For this review, use the dimensioned drawing (mm, ordinates from the lowest corner) and the shaded views. A direction names the side the tool comes from. Give positions to 0.01 mm unless a question says otherwise; leave off trailing zeros. Order: outer loops, then holes, each group sorted by start corner. A loop starts at its lowest first (then second) coordinate and runs counter-clockwise, first axis right, second up. Notation, with made-up numbers: (30.25, 58.5) -> (85.25, 58.5) arc R22 cw to (85.25, 67.5) -> close; hole circle Ø9 at (85.5, 85). An arc over 180 degrees is marked (long way). Answer as a JSON object with one key per item and string values. Group by question number.
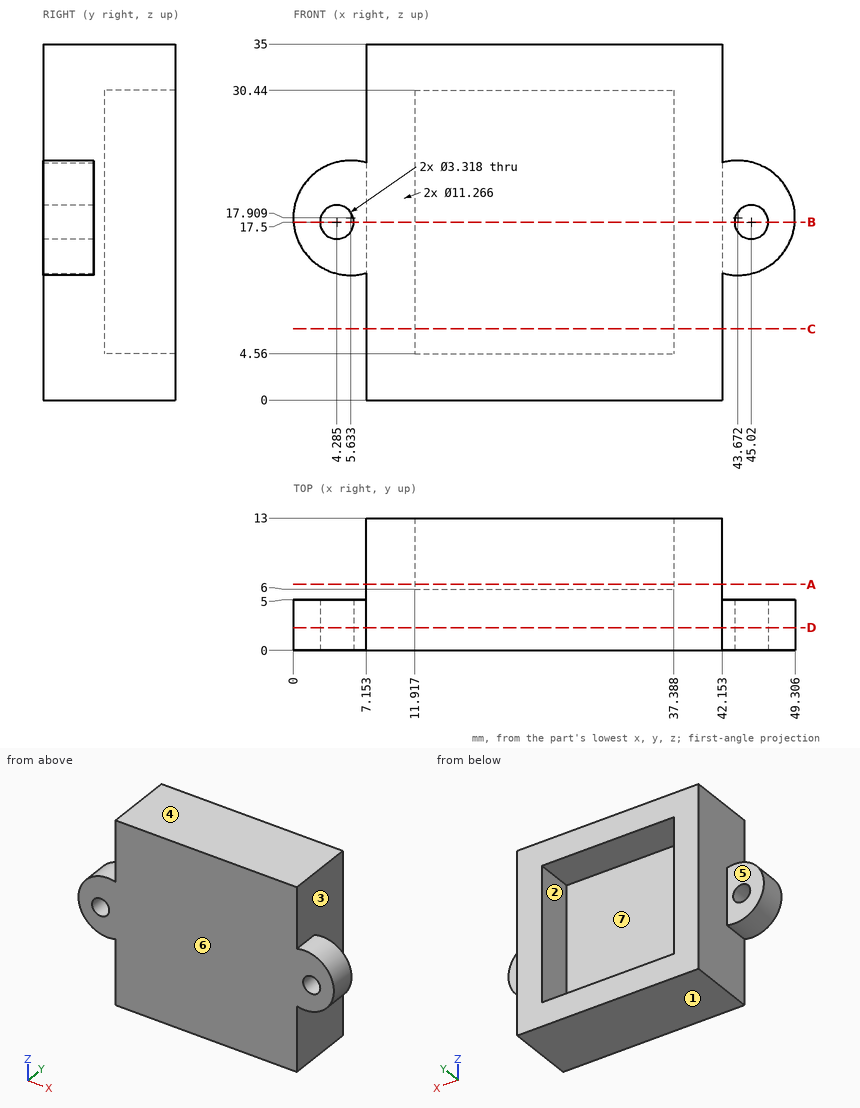
1. For probe 1 along Z at (x, y) = (37, 6.25); probe 2 along X at (y, z) = (7.5, 17.5); probe 3 along X at (y, z) = (2.55, 17.5) (1 decimal), list the stretches that pass through material, from the lowest coordinate up. Write a range as [from, to].
2. Machinability: for the marked faces 5, 6 and 7, which of the approach directions +Z, -Z, +X, -X, +Y, -Y give a long, thin tool a straight path to every point of the face, cutting with its end or side? Answer none if there is none.
3. For pin 1 (7.5 mm diameter, centred on y = 9, z = 13.5, fed in from -X); pin 2 (7.5 mm diameter, centred on y = 10.5, z = 11.5, fed in from +X), all flat-tipped, find the tip position at first contact; note any pin that passes through.
4. Take a section at B-B on z = 17.5. Give the boundary of the cut face in (x, y) (1 decimal).
5. Take a section at C-C on z = 7. Give the boundary of the cut face in (x, y).
6. Draft analysis for pull direction Z (two halves, no side actions). For the marked faces 1, 2, 3 and 4, state which applies: pulls with the +Z half, pulls with the -Z half, needs draft (parallel to the pull), parting line crosses it, or undercut.
7. Take a section at A-A on y = 6.5. Give the boundary of the cut face in (x, z).
8. Take a section at D-D on y = 2.25. Give the boundary of the cut face in (x, z) (1 decimal), plus the area to 3 significant figures.
Checks:
{
 "1": {"probe 1": "z = [0, 4.56], [30.44, 35]", "probe 2": "x = [7.15, 11.92], [37.39, 42.15]", "probe 3": "x = [0, 2.6], [5.9, 43.4], [46.7, 49.3]"},
 "2": {"face 5": "+Z, -Z, -X, +Y", "face 6": "+Z, -Z, +X, -X, -Y", "face 7": "+Y"},
 "3": {"pin 1": "stops at x = 7.15", "pin 2": "stops at x = 42.15"},
 "4": {"outline": "(0, 0) -> (2.6, 0) -> (2.6, 5) -> (0, 5) -> close; (5.9, 0) -> (43.4, 0) -> (43.4, 5) -> (42.2, 5) -> (42.2, 13) -> (37.4, 13) -> (37.4, 6) -> (11.9, 6) -> (11.9, 13) -> (7.2, 13) -> (7.2, 5) -> (5.9, 5) -> close; (46.7, 0) -> (49.3, 0) -> (49.3, 5) -> (46.7, 5) -> close"},
 "5": {"outline": "(7.15, 0) -> (42.15, 0) -> (42.15, 13) -> (37.39, 13) -> (37.39, 6) -> (11.92, 6) -> (11.92, 13) -> (7.15, 13) -> close"},
 "6": {"face 1": "pulls with the -Z half", "face 2": "undercut", "face 3": "needs draft", "face 4": "pulls with the +Z half"},
 "7": {"outline": "(7.15, 0) -> (42.15, 0) -> (42.15, 35) -> (7.15, 35) -> close; hole (11.92, 4.56) -> (37.39, 4.56) -> (37.39, 30.44) -> (11.92, 30.44) -> close"},
 "8": {"outline": "(7.2, 0) -> (42.2, 0) -> (42.2, 12.5) arc R5.6 ccw (long way) to (42.2, 23.3) -> (42.2, 35) -> (7.2, 35) -> (7.2, 23.3) arc R5.6 ccw (long way) to (7.2, 12.5) -> close; hole circle Ø3.3 at (4.3, 17.5); hole circle Ø3.3 at (45, 17.5)", "area": "1,340 mm2"}
}
